Geometry: see drawing. Coordinates: mm, zero at the bounding-box minimum. Round coordinates to 2 decimals unless told otherwise and drop trailing zeros. Loops run counter-clockwise (first coordinate to the right, second up) from the corner with the lowest first, then second, coordinate; pieces in that order, holes last.
(1) Cut plane B-B, the plane x = 65. Output: boundary loops of the cut face in (y, z), and give its area (3 significant figures).
(2) Line query: line 1 (Y direction, x = 95, z = 1.6); line 2 (Y direction, x = 76.5, z = 2.7); line 3 (X direction, y = 121, z = 1.15). Output: solid intervals per line, ascending.
(3) Cut plane A-A, the plane y = 95. Output: boundary loops of the cut face in (x, z), and give its area (3 significant figures).
(4) Cut plane C-C, the plane z = 0.6. Output: boundary loops of the cut face in (x, y), and give its area (3 significant figures).
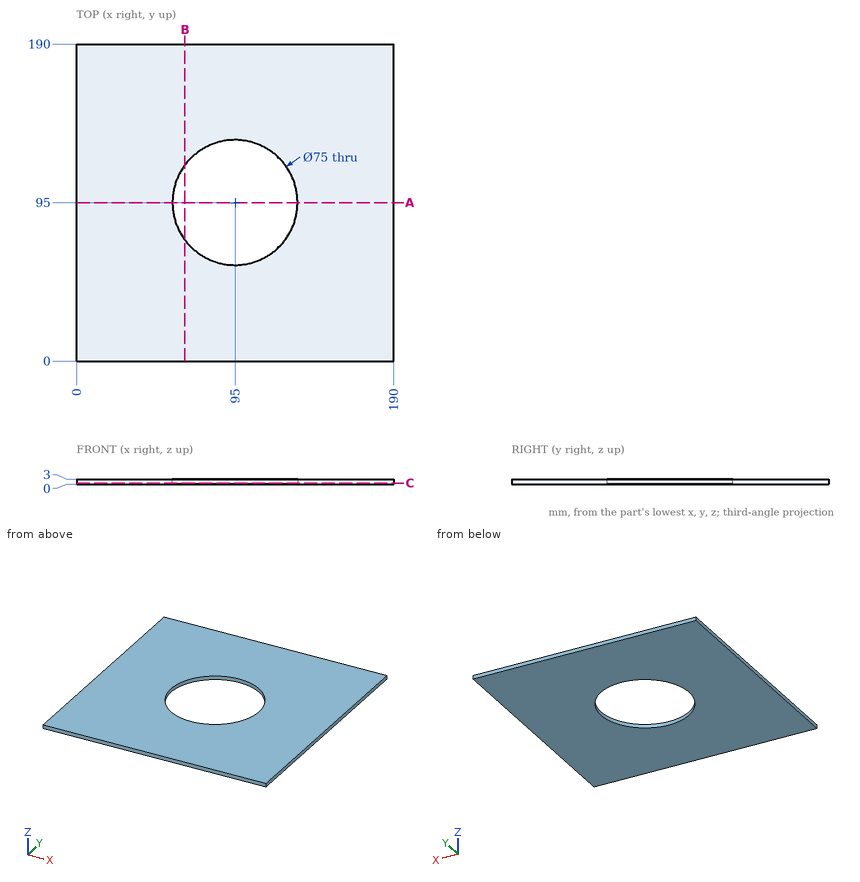
Reported:
1. outline: (0, 0) - (72.5, 0) - (72.5, 3) - (0, 3) - close; (117.5, 0) - (190, 0) - (190, 3) - (117.5, 3) - close
1. area: 435 mm2
2. line 1: y = 0 to 57.5, 132.5 to 190
2. line 2: y = 0 to 62.38, 127.62 to 190
2. line 3: x = 0 to 67.98, 122.02 to 190
3. outline: (0, 0) - (57.5, 0) - (57.5, 3) - (0, 3) - close; (132.5, 0) - (190, 0) - (190, 3) - (132.5, 3) - close
3. area: 345 mm2
4. outline: (0, 0) - (190, 0) - (190, 190) - (0, 190) - close; hole circle Ø75 at (95, 95)
4. area: 31,700 mm2
